Print and shaded views of the part. All mm, measured from the part's lowest x, y and z. Round coordinates to 2 decimals unless told otherwise and drop trailing zeros. Loops run counter-clockwise (first coordinate to the right, second up) from the corner with the lowest first, then second, coordinate; pieces in that order, holes last. Notation, with made-up numbers: (35.5, 39) - (51.5, 39) arc R3 cw to (51.5, 43) - close; hole circle Ø8 at (68.25, 34.5). An arc over 180 degrees is marked (long way). Use one line per item in the form item = value.
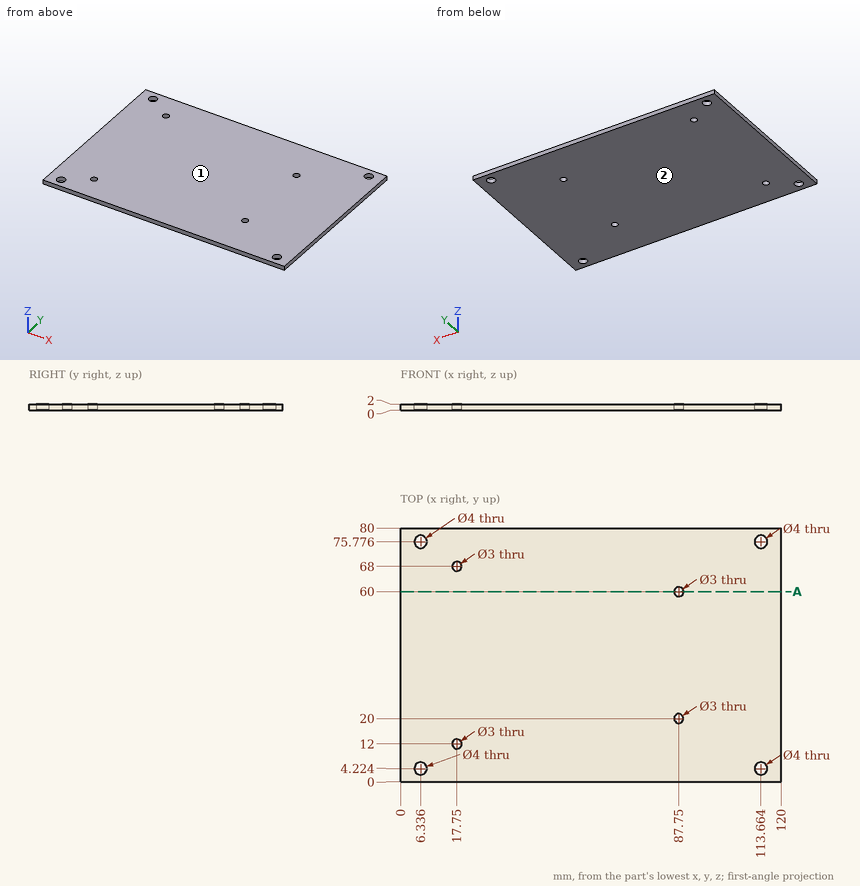
1) Drill centre lines: probe 1 along Y at (x, z) = (88, 0.75); probe 2 along Y at (x, z) = (17.75, 1.3); probe 3 along X at (y, z) = (76, 1.9). Where is each one in solid material? Low to high.
Report:
probe_1 = 0 to 18.52, 21.48 to 58.52, 61.48 to 80
probe_2 = 0 to 10.5, 13.5 to 66.5, 69.5 to 80
probe_3 = 0 to 4.35, 8.32 to 111.68, 115.65 to 120
2) Slice it at A-A (y = 60). Write the cut outline in (x, z), plus the area to 3 significant figures.
Report:
outline = (0, 0) - (86.25, 0) - (86.25, 2) - (0, 2) - close; (89.25, 0) - (120, 0) - (120, 2) - (89.25, 2) - close
area = 234 mm^2
3) Two-plate mould, pull along Z, no slides. Class the marked faces 1 and 2: +Z half, -Z half, draft (parallel to the pull), parting line (faces both ways), or undercut.
Report:
face_1 = +Z half
face_2 = -Z half
